```python
from build123d import *

# Parameters (mm, degrees)
F1_DEPTH = 2


with BuildPart() as f1:
    # F0 (on Top) → F1 (new body, symmetric)
    with BuildSketch(Plane.XY):
        Polygon((0, 91.5), (0, 0), (0, -91.5), (58, -91.5), (58, -39.5), (133, -39.5), (133, -91.5), (268, -91.5), (268, -39.5), (343, -39.5), (343, -91.5), (350, -91.5), (400, -41.5), (400, 0), (400, 41.5), (350, 91.5), (343, 91.5), (343, 39.5), (268, 39.5), (268, 91.5), (133, 91.5), (133, 39.5), (58, 39.5), (58, 91.5), align=None)
    extrude(amount=F1_DEPTH, both=True)


solid = f1.part
```
Design review of the part built by this model. Coordinates are the model's own, in mm. Coordinates: 2 decimals unless noted, no trailing zeros. Loops run counter-clockwise (first coordinate to the right, second up) from the corner with the lowest first, then second, coordinate; pieces in that order, holes last. Notation, with made-up numbers: M 18,54.5 L 61,54.5 A24 ccw 61,80.5 Z; hole C 31,81.25 d11. An arc over 180 degrees is marked long. One line per question, with ' | ' between items.
(1) We need section A-A (y = -69). Give the boundary of the cut face in (x, z).
Filled in:
outline: M 0,-2 L 58,-2 L 58,2 L 0,2 Z; M 133,-2 L 268,-2 L 268,2 L 133,2 Z; M 343,-2 L 372.5,-2 L 372.5,2 L 343,2 Z
(2) We need section B-B (y = -46). Give the boundary of the cut face in (x, z), and give its area (3 significant figures).
Filled in:
outline: M 0,-2 L 58,-2 L 58,2 L 0,2 Z; M 133,-2 L 268,-2 L 268,2 L 133,2 Z; M 343,-2 L 395.5,-2 L 395.5,2 L 343,2 Z | area: 982 mm^2
(3) Wall thickness on probe 1 along X at (y, z) = (76, -1.35); probe 2 along X at (y, z) = (70, -0.45); probe 3 along Y at (x, z) = (96.5, -1.3): over which ranges is each line inside the solid? List them lowest first.
Filled in:
probe 1: x = 0 to 58, 133 to 268, 343 to 365.5 | probe 2: x = 0 to 58, 133 to 268, 343 to 371.5 | probe 3: y = -39.5 to 39.5
(4) For pin 1 Ø2 at (x, z) = (101, -1) entering from -Y; pin 2 Ø1.2 at (x, z) = (92, 0) entering from +Y; pin 3 Ø1.2 at (y, z) = (-74.5, -1) entering from +X, all flat-tipped, find the tip position at first contact; note any pin that passes through.
Filled in:
pin 1: stops at y = -39.5 | pin 2: stops at y = 39.5 | pin 3: stops at x = 367.6
(5) We need section D-D (x = 299). Give the boundary of the cut face in (y, z).
Filled in:
outline: M -39.5,-2 L 39.5,-2 L 39.5,2 L -39.5,2 Z
(6) We need section C-C (z = 1.4). Give the boundary of the cut face in (x, y), and give its area (3 significant figures).
Filled in:
outline: M 0,-91.5 L 58,-91.5 L 58,-39.5 L 133,-39.5 L 133,-91.5 L 268,-91.5 L 268,-39.5 L 343,-39.5 L 343,-91.5 L 350,-91.5 L 400,-41.5 L 400,41.5 L 350,91.5 L 343,91.5 L 343,39.5 L 268,39.5 L 268,91.5 L 133,91.5 L 133,39.5 L 58,39.5 L 58,91.5 L 0,91.5 Z | area: 55,100 mm^2
